Study the drawing (mm; zero at the part's minimum x, y, z) and answer. A direction names the side the tool comes from. Round coordinates to 2 decimals unless told otherwise and drop trailing zeros. Write each loop counter-clockwise with the first axis right and the second up, starting at its lowest first coordinate (ties: lowest second). Pieces come first, ordered by that corner, then holes. Notation, with made-up numbers: (20.5, 61) -> (40.5, 61) arc R18 cw to (40.5, 89) -> close; hole circle Ø8 at (51.25, 63.25). An arc over 180 degrees is marked (long way). One line per question, with ' | ' between items. Start each with the question number.
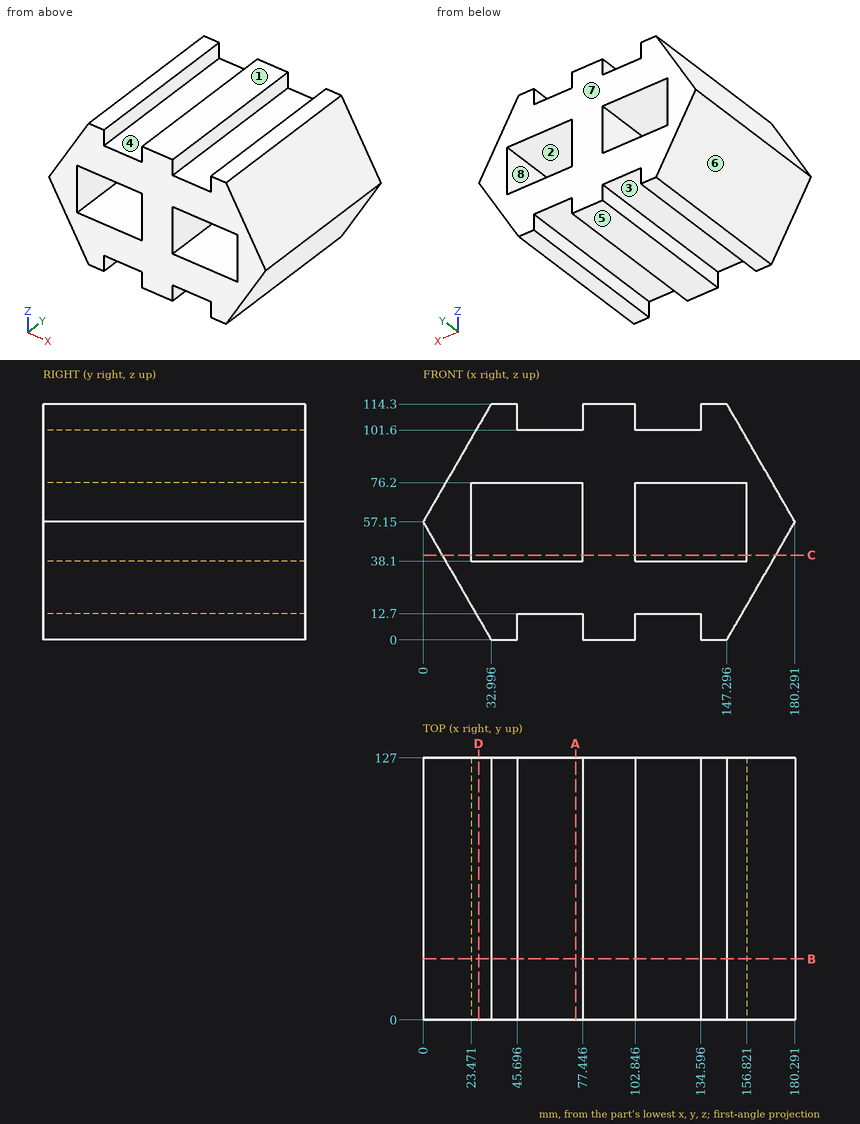
(1) The mould has two halves that part along Z. Classify the marked faces 6, 7 and 8: +Z half, -Z half, draft (parallel to the pull), parting line (faces both ways), or undercut.
(2) A cutting plane is placed at B-B, the plane y = 29.5. Count the separate pieces of the cut face and the enclosed holes in it, then the cut area to 3 significant figures.
(3) Consider L1, parallel to Z at x = 147, y = 62; L2, parallel to X at y = 45.5, z = 60 (1 decimal); L3, parallel to X at y = 118.5, z = 45 (1 decimal). Determine where each line is inside the solid, lowest interval first.
(4) For the marked faces 1, 2, 3, 4 and 5, determine the directions among +Z, -Z, +X, -X, +Y, -Y from which every point of the face is accessible in a straight line to the end or side of a thin tool.
(5) A cutting plane is placed at C-C, the plane z = 41. Determine the outline of the cut face in (x, y) (1 decimal).
(6) A cutting plane is placed at A-A, the plane x = 74. Determine the outline of the cut face in (y, z), then the cut area to 3 significant figures.
(7) A cutting plane is placed at D-D, the plane x = 27. Determine the outline of the cut face in (y, z) (1 decimal).
(8) Given pin 1 Ø6.5 at (y, z) = (70.5, 108) entering from +X; pin 2 Ø10 at (y, z) = (82, 111) entering from +X; pin 3 Ø11.5 at (y, z) = (34.5, 56.5) entering from +X, each flat-ended and moving along its own axis, determine where each tip first touches the part or whether it passes through.
Returned:
1) face 6: -Z half | face 7: draft | face 8: undercut
2) separate pieces: 1 | enclosed holes: 2 | area: 11,100 mm2
3) L1: 0 to 38.1, 76.2 to 114.3 | L2: 1.6 to 23.5, 77.4 to 102.8, 156.8 to 178.6 | L3: 7 to 23.5, 77.4 to 102.8, 156.8 to 173.3
4) face 1: +Z, +X, -X, +Y, -Y | face 2: +Y, -Y | face 3: -Z, +Y, -Y | face 4: +Z, +Y, -Y | face 5: -Z, +X, -X, +Y, -Y
5) outline: (9.3, 0) -> (23.5, 0) -> (23.5, 127) -> (9.3, 127) -> close; (77.4, 0) -> (102.8, 0) -> (102.8, 127) -> (77.4, 127) -> close; (156.8, 0) -> (171, 0) -> (171, 127) -> (156.8, 127) -> close
6) outline: (0, 12.7) -> (127, 12.7) -> (127, 38.1) -> (0, 38.1) -> close; (0, 76.2) -> (127, 76.2) -> (127, 101.6) -> (0, 101.6) -> close | area: 6,450 mm2
7) outline: (0, 10.4) -> (127, 10.4) -> (127, 38.1) -> (0, 38.1) -> close; (0, 76.2) -> (127, 76.2) -> (127, 103.9) -> (0, 103.9) -> close
8) pin 1: x = 152.81 | pin 2: x = 152.09 | pin 3: x = 180.29
